Geometry: see drawing. Coordinates: mm, zero at the bounding-box minimum. A direction names the side the tool comes from. Give positions to 0.01 mm unless a question says otherwise; leave off trailing zeros. Loops run counter-clockwise (first coordinate to the right, second up) from the corner with the lowest first, then second, coordinate; pieces in that order, holes last. Notation, with made-up numbers: (68, -24) -> (72, -24) arc R6 ccw to (72, -16) -> close; hole circle Ø8 at (61.25, 63.25). An arc over 180 degrees is marked (long way). Use CSV: the item, a comma, the result in double quotes.
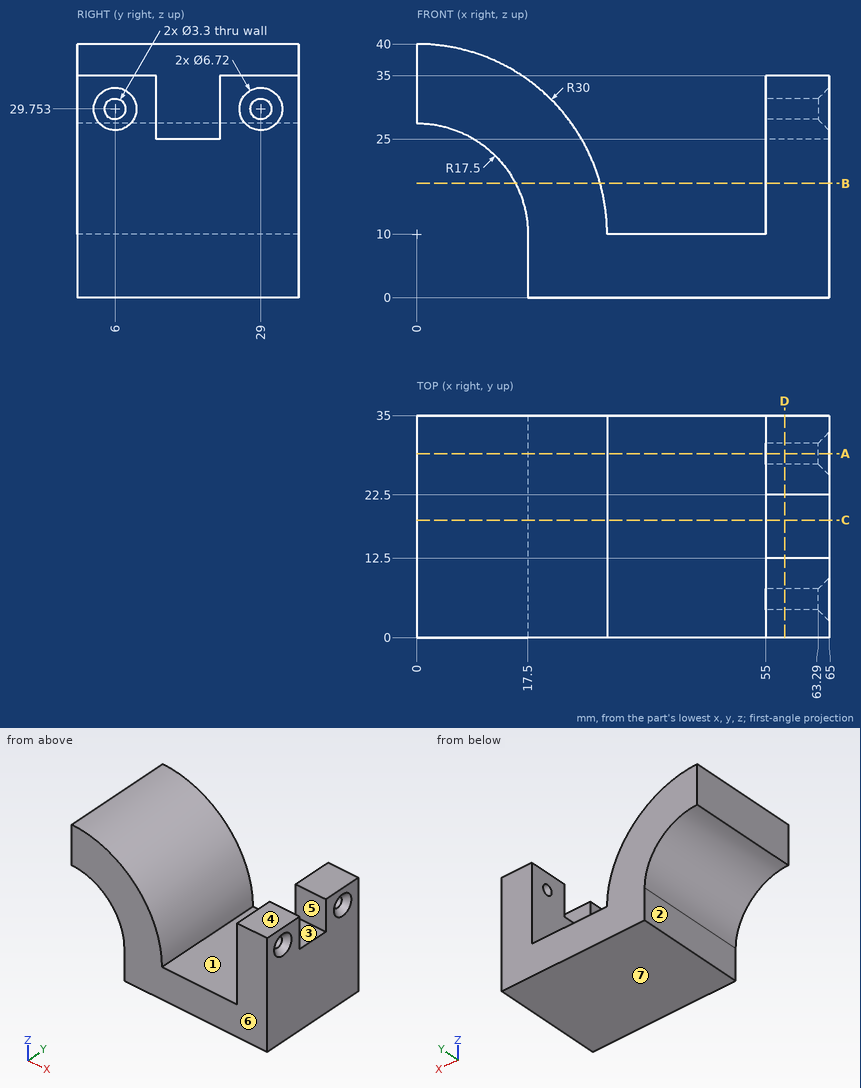
1) Mould query, pull axis Y, two halves, no side actions, for the marked faces 5, 6 and 7. Classes: pulls with the +Y half, pulls with the -Y half, needs draft (parallel to the pull), parting line crosses it, or undercut.
From the geometry:
face 5,"undercut"
face 6,"pulls with the -Y half"
face 7,"needs draft"
2) Section query A-A (y = 29). Return loops of the section in (x, z).
From the geometry:
outline,"(0, 27.5) arc R17.5 cw to (17.5, 10) -> (17.5, 0) -> (65, 0) -> (65, 26.39) -> (63.29, 28.1) -> (55, 28.1) -> (55, 10) -> (30, 10) arc R30 ccw to (0, 40) -> close; (55, 31.4) -> (63.29, 31.4) -> (65, 33.11) -> (65, 35) -> (55, 35) -> close"
3) Section query C-C (y = 18.5). Return loops of the section in (x, z), then the cut area to 3 significant figures.
From the geometry:
outline,"(0, 27.5) arc R17.5 cw to (17.5, 10) -> (17.5, 0) -> (65, 0) -> (65, 25) -> (55, 25) -> (55, 10) -> (30, 10) arc R30 ccw to (0, 40) -> close"
area,"1,090 mm^2"
4) Ray query, line 1 (Z direction, x = 58.75, y = 6); line 2 (X direction, y = 6.5, z = 10.5); line 3 (Z direction, x = 47, y = 19.5). Return the intervals inside material, ascending.
From the geometry:
line 1,"z = 0 to 28.1, 31.4 to 35"
line 2,"x = 17.49 to 30, 55 to 65"
line 3,"z = 0 to 10"
5) Section query B-B (z = 18). Return loops of the section in (x, y), then the cut area to 3 significant figures.
From the geometry:
outline,"(15.56, 0) -> (28.91, 0) -> (28.91, 35) -> (15.56, 35) -> close; (55, 0) -> (65, 0) -> (65, 35) -> (55, 35) -> close"
area,"817 mm^2"
6) Contact query for flat-ended pins moving along their axis: pin 1 (3 mm diameter, centred on y = 25, z = 5.5, fed in from -X); pin 2 (2 mm diameter, centred on y = 6, z = 29.75, fed in from +X); pin 3 (12 mm diameter, centred on x = 7, y = 24, fed in from +Z). Output: stop coordinate, or through.
From the geometry:
pin 1,"stops at x = 17.5"
pin 2,"stops at x = 23.42"
pin 3,"stops at z = 39.98"
7) Reachability of the marked faces 1, 2, 3 and 4 from +Z, -Z, +X, -X, +Y, -Y: full face, straight path, thin tool, end or side. Return the list, or none.
From the geometry:
face 1,"+Z, +Y, -Y"
face 2,"-Z, -X, +Y, -Y"
face 3,"+Z, +X"
face 4,"+Z, +X, +Y, -Y"
8) Section query D-D (x = 58). Return loops of the section in (y, z).
From the geometry:
outline,"(0, 0) -> (35, 0) -> (35, 35) -> (22.5, 35) -> (22.5, 25) -> (12.5, 25) -> (12.5, 35) -> (0, 35) -> close; hole circle Ø3.3 at (6, 29.75); hole circle Ø3.3 at (29, 29.75)"
